Study the drawing (mm; zero at the part's minimum x, y, z) and answer. A direction names the side the tool comes from. Coordinates: 2 decimals unless noted, no trailing zeros. Order: outer loops, then holes, each group sorted by start corner. A loop starts at its lowest first (then second) coordinate and runs counter-clockwise, first axis right, second up. Notation, with made-up numbers: (40, 55) -> (76, 55) arc R8 cw to (76, 59) -> close; hole circle Ø2 at (22, 45). An arc over 180 degrees is marked (long way). Write each question's results on one line, items separated by ' | '. Start each with the question number.
(1) The part is cut by section B-B, the plane x = 9.85. Give the vertices of the cut face in (y, z), then the cut area to 3 significant figures.
(2) Given pin 1 (2.5 mm diameter, centred on x = 2.5, z = 5.5, fed in from -Y); pin 2 (1.5 mm diameter, centred on y = 4, z = 14, fed in from -X); pin 3 (2.5 mm diameter, centred on x = 16, z = 6, fed in from -Y), each flat-ended and moving along its own axis, determine where each tip first touches the part or whether it passes through.
(3) Determine the mould class of the marked faces 3 and 4 for opening direction Y: +Y half, -Y half, draft (parallel to the pull), parting line (faces both ways), or undercut.
(4) The part is cut by section D-D, the plane y = 4.5. Give the vertices of the cut face in (x, z), then the cut area to 3 significant figures.
(5) The part is cut by section C-C, the plane z = 19.5. Give the vertices of the cut face in (x, y), then the cut area to 3 significant figures.
(6) The part is cut by section A-A, the plane z = 6. Give the vertices of the cut face in (x, y).
(7) Straight lines are drawn through the part: L1, parallel to Z at x = 12.5, y = 10.5; L2, parallel to Y at x = 8.75, z = 6.5; L3, parallel to Y at x = 18.5, z = 16.5. For each, find the intervals that lie inside material, in ascending order.
(8) A tool of negligible diameter and unlimited length cuts with its end or side. For the marked faces 1 and 2, from which of +Z, -Z, +X, -X, +Y, -Y can it reach the whole face along a straight path? Write none if from no direction.
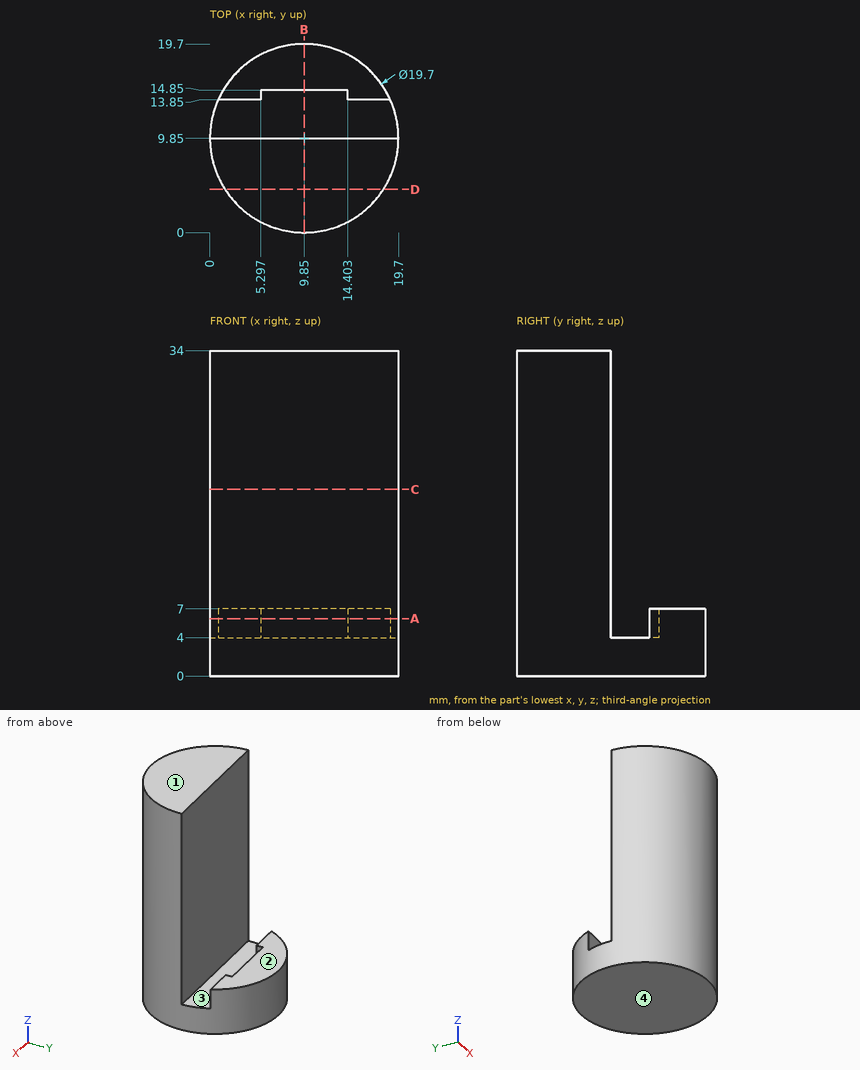
Established:
1) outline: (0, 0) -> (19.7, 0) -> (19.7, 7) -> (14.85, 7) -> (14.85, 4) -> (9.85, 4) -> (9.85, 34) -> (0, 34) -> close | area: 389 mm^2
2) pin 1: stops at y = 2.12 | pin 2: stops at x = 1.42 | pin 3: stops at y = 1.31
3) face 3: undercut | face 4: draft
4) outline: (1.58, 0) -> (18.12, 0) -> (18.12, 34) -> (1.58, 34) -> close | area: 562 mm^2
5) outline: (0, 9.85) arc R9.85 ccw to (19.7, 9.85) -> close | area: 152 mm^2
6) outline: (0, 9.85) arc R9.85 ccw to (19.7, 9.85) -> close; (0.85, 13.85) -> (5.3, 13.85) -> (5.3, 14.85) -> (14.4, 14.85) -> (14.4, 13.85) -> (18.85, 13.85) arc R9.85 ccw to start
7) L1: z = 0 to 4 | L2: y = 0.06 to 9.85, 14.85 to 19.64 | L3: y = 5.14 to 9.85
8) face 1: +Z, +X, -X, +Y, -Y | face 2: +Z, +X, -X, +Y
